Model file for the job. Use its own axes, mm. A direction names the side the tool comes from. Coordinates: 2 decimals unless noted, no trailing zeros. Order: outer loops, then holes, each group sorted by start corner. A loop starts at its lowest first (then second) coordinate and runs counter-clockwise, first axis right, second up. Notation, with made-up numbers: (10, 61) -> (56, 61) arc R15 ccw to (56, 74) -> close; hole circle Ø1 at (22.5, 0.25). An arc over 180 degrees is marked (long way). Write item = value, one per line. Start each with the question number.
Q1. Cut at A-A, the plane x = 0. List the corners of the cut face in (y, z), plus the area to 3 significant figures.
Q2. Mould opens along Y. For faces 1 (the face through (0, 74, 0)), 2 (the face through (-10, 64, 3)), 3 (the face through (0.66, 67.944, -14.985)), 4 (the face through (0.96, 9.31, -0.14)) say: +Y half, -Y half, draft (parallel to the pull), parting line (faces both ways), or undercut.
Q3. Wall check: line 1 (Y direction, x = 0, z = -3.5); line 2 (Y direction, x = -7.25, z = -8); line 3 (X direction, y = 7, z = -0.5). Give the ranges that are in metal, low to high. Write a range as from..to.
Q4. 3-axis set-ups, long thin cutter, end or side, ignore diameter. For faces 5 (the face through (0, 0, 0)), 6 (the face through (3, 32.57, 9.54)): which of +Z, -Z, +X, -X, +Y, -Y reach the whole face in a straight line?
Q5. Flat gauge pins, fed straight in: pin 1 (8 mm diameter, centred on y = 58, z = -7, fed in from +X); pin 2 (2 mm diameter, centred on x = -8, y = 16, fed in from -Z); pin 3 (4.5 mm diameter, centred on x = 0, y = 7, fed in from -Z); pin 4 (5 mm diameter, centred on x = -1, y = 44.5, fed in from -Z). Where does each tip first touch, or does it go through?
Q6. Cut at C-C, the plane y = 7. List the corners of the cut face in (x, z), plus the area to 3 significant figures.
Q7. Cut at B-B, the plane z = 0. List the corners of the cut face in (x, y).
from build123d import *

# Parameters (mm, degrees)
SKETCH1_R               = 10
BOSS_EXTRUDE1_DEPTH     = 64
SKETCH2_R               = 15
BOSS_EXTRUDE2_DEPTH     = 10
CUT_EXTRUDE1_DEPTH      = 77.980517016
CUT_EXTRUDE1_DEPTH_BACK = 77.980517016
SKETCH3_R               = 2.5
FILLET1_R               = 2


with BuildPart() as part:
    # Sketch1 → Boss-Extrude1 (new body)
    with BuildSketch(Plane(origin=(0, 0, 0), x_dir=(1, 0, 0), z_dir=(0, 1, 0))):
        with Locations(Location((0, 0, 0), (0, 0, 270))):
            Circle(SKETCH1_R)
    extrude(amount=BOSS_EXTRUDE1_DEPTH)

    # Sketch2 → Boss-Extrude2 (add)
    with BuildSketch(Plane(origin=(0, 64, 0), x_dir=(1, 0, 0), z_dir=(0, 1, 0))):
        with Locations(Location((0, 0, 0), (0, 0, 270))):
            Circle(SKETCH2_R)
    extrude(amount=BOSS_EXTRUDE2_DEPTH)

    # Sketch3 → Cut-Extrude1 (cut, two sides: drawn at the far end of the back side and taken through both)
    with BuildSketch(Plane.XY.offset(-CUT_EXTRUDE1_DEPTH_BACK)):
        with Locations(Location((0, 7, 0), (0, 0, 90.000000004))):
            Circle(SKETCH3_R)
    extrude(amount=CUT_EXTRUDE1_DEPTH + CUT_EXTRUDE1_DEPTH_BACK, mode=Mode.SUBTRACT)

    # Fillet1
    fillet1_edges = [part.edges().sort_by_distance(p)[0] for p in [
        (0, 0, -10),
        (0, 74, -15),
    ]]
    fillet(fillet1_edges, radius=FILLET1_R)


solid = part.part
Here are the results:
q1.outline = (0, -8) arc R2 ccw to (2, -10) -> (4.5, -10) -> (4.5, 10) -> (2, 10) arc R2 ccw to (0, 8) -> close; (9.5, -10) -> (64, -10) -> (64, -15) -> (72, -15) arc R2 ccw to (74, -13) -> (74, 13) arc R2 ccw to (72, 15) -> (64, 15) -> (64, 10) -> (9.5, 10) -> close
q1.area = 1,480 mm²
q2.face_1 = +Y half
q2.face_2 = -Y half
q2.face_3 = draft
q2.face_4 = undercut
q3.line_1 = 0..4.5, 9.5..74
q3.line_2 = 64..74
q3.line_3 = -9.99..-2.5, 2.5..9.99
q4.face_5 = +Z, -Z, +X, -X, -Y
q4.face_6 = -Y
q5.pin_1 = 9.54
q5.pin_2 = -7.14
q5.pin_3 = through
q5.pin_4 = -10
q6.outline = (-2.5, -9.68) -> (-2.5, 9.68) arc R10 ccw to start; (2.5, -9.68) arc R10 ccw to (2.5, 9.68) -> close
q6.area = 215 mm²
q7.outline = (-15, 64) -> (-10, 64) -> (-10, 2) arc R2 ccw to (-8, 0) -> (8, 0) arc R2 ccw to (10, 2) -> (10, 64) -> (15, 64) -> (15, 72) arc R2 ccw to (13, 74) -> (-13, 74) arc R2 ccw to (-15, 72) -> close; hole circle Ø5 at (0, 7)
